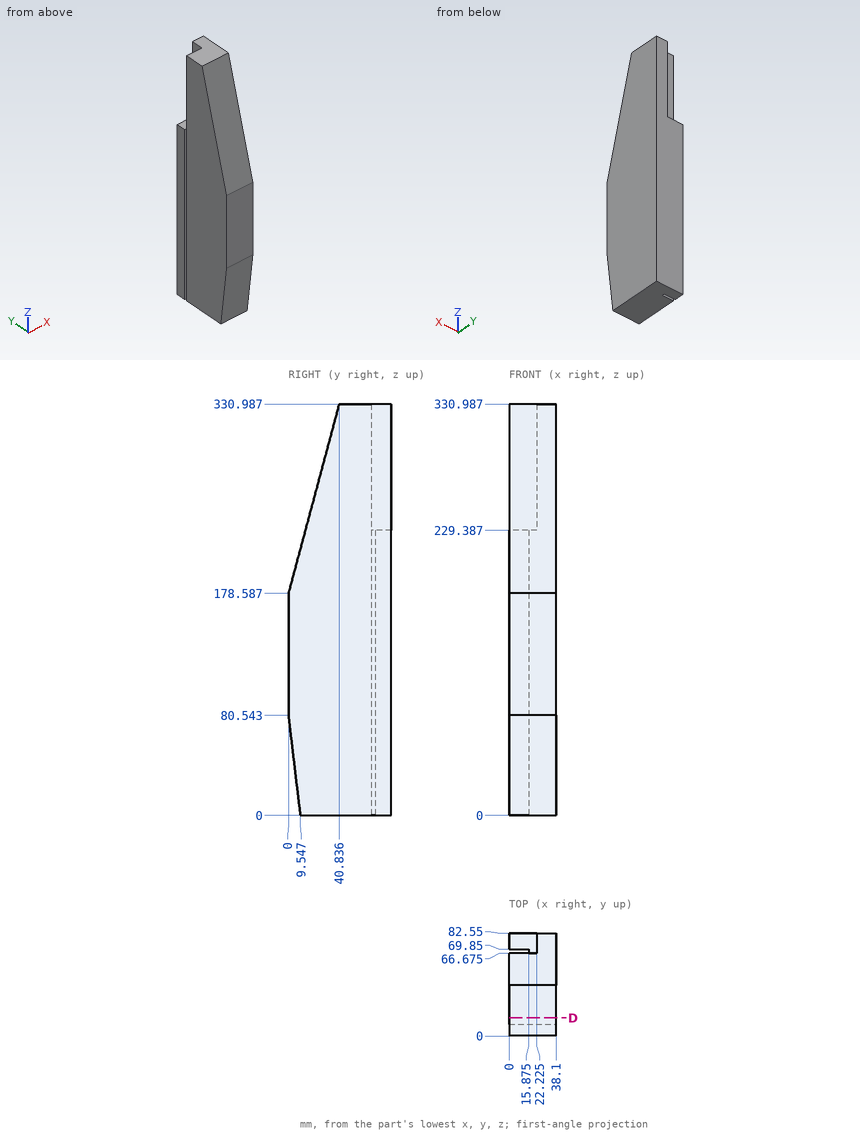
Source: three-view drawing plus pictorial views. Frame: mm from the lowest corner of the part. Coordinates: 2 decimals unless noted, no trailing zeros. Loops run counter-clockwise (first coordinate to the right, second up) from the corner with the lowest first, then second, coordinate; pieces in that order, holes last. Notation, with made-up numbers: (-16, 48) - (27, 48) arc R18 cw to (27, 64) - close; hole circle Ø5 at (81.25, -5). An arc over 180 degrees is marked (long way). Answer in a Markdown table with one row per item. Add a question column.
Item 1: Line query: line 1 along Z through (x, y) = (10.5, 71); line 2 along X through (y, z) = (67.5, 190) (1 decimal); line 3 along Y through (x, z) = (5, 245.5) (1 decimal). Output: solid intervals per line, ascending. Write a range as [from, to].
Item 2: Section query D-D on y = 14.5. Return the cut outline in (x, z), then the cut area to 3 significant figures.
Item 3: Contact query for flat-ended pins moving along their axis: P1, Ø12.5, axis at y = 72, z = 287.5, coming from the -X side; P2, Ø1, axis at y = 69, z = 119.5, coming from the -X side (1 decimal); P3, Ø12.5, axis at x = 15.5, y = 76.5, coming from the +Z side; P4, Ø5, axis at x = 25.5, z = 187.5, coming from the -Y side. Output: stop coordinate, or through.
Recorded:
| question | item | result |
|---|---|---|
| 1 | line 1 | [0, 229.39] |
| 1 | line 2 | [15.9, 38.1] |
| 1 | line 3 | [17.9, 66.7] |
| 2 | outline | (0, 0) - (38.1, 0) - (38.1, 232.7) - (0, 232.7) - close |
| 2 | area | 8,870 mm^2 |
| 3 | P1 | x = 0 |
| 3 | P2 | x = 15.9 |
| 3 | P3 | z = 229.39 |
| 3 | P4 | y = 1.72 |
